Autodesk Fusion 360 part; units mm, degrees
sketch "Sketch1" plane through (0, 0, 0) normal (0, 0, 1) x (1, 0, 0)
  line L0 (18.75, -9.5) -> (-18.75, -9.5)
  line L1 (-18.75, -9.5) -> (-18.75, 9.5)
  line L2 (-18.75, 9.5) -> (18.75, 9.5)
  line L3 (18.75, 9.5) -> (18.75, -9.5)
  line L4 (18.75, -9.5) -> (-18.75, 9.5) construction
  line L5 (-18.75, -9.5) -> (18.75, 9.5) construction
  line L6 (0, 9.5) -> (0, -9.5) construction
  line L7 (12.7, 9.5) -> (12.7, -9.5) construction
  line L8 (-12.7, 9.5) -> (-12.7, -9.5) construction
  line L9 (-5.1, -7.1) -> (3, -7.1)
  line L10 (-3.1043, 7.1) -> (4.9957, 7.1)
  line L11 (-5.1, -7.1) -> (-3.1043, 7.1)
  line L12 (3, -7.1) -> (4.9957, 7.1)
  line L13 (-1.9308, 5.75) -> (3.4427, 5.75)
  line L14 (1.8265, -5.75) -> (3.4427, 5.75)
  line L15 (-3.547, -5.75) -> (1.8265, -5.75)
  line L16 (-3.547, -5.75) -> (-1.9308, 5.75)
  line L17 (-17.8, -7.1) -> (-15.8043, 7.1)
  line L18 (-16.247, -5.75) -> (-14.6308, 5.75)
  line L19 (-17.8, -7.1) -> (-9.7, -7.1)
  line L20 (-16.247, -5.75) -> (-10.8735, -5.75)
  line L21 (-10.8735, -5.75) -> (-9.2573, 5.75)
  line L22 (-9.7, -7.1) -> (-7.7043, 7.1)
  line L23 (-14.6308, 5.75) -> (-9.2573, 5.75)
  line L24 (-15.8043, 7.1) -> (-7.7043, 7.1)
  line L25 (7.6, -7.1) -> (9.5957, 7.1)
  line L26 (9.153, -5.75) -> (10.7692, 5.75)
  line L27 (7.6, -7.1) -> (15.7, -7.1)
  line L28 (9.153, -5.75) -> (14.5265, -5.75)
  line L29 (14.5265, -5.75) -> (16.1427, 5.75)
  line L30 (15.7, -7.1) -> (17.6957, 7.1)
  line L31 (10.7692, 5.75) -> (16.1427, 5.75)
  line L32 (9.5957, 7.1) -> (17.6957, 7.1)
  dimension "d1" = 37.5
  dimension "d2" = 19
  dimension "d3" = 12.7
  dimension "d4" = 12.7
  dimension "d5" = 8.1
  dimension "d6" = 3
  dimension "d7" = 2.4
  dimension "d8" = 8.1
  dimension "d9" = 2.4
  dimension "d10" = 82
  dimension "d11" = -1.35
  dimension "d14" = 12.7
  dimension "d15" = 0
extrude "Extrude1" add sketch "Sketch1" against normal blind 8 contours L0 L1 L2 L3 | L9 L10 L11 L12 | L13 L14 L15 L16 | L17 L19 L22 L24 | L18 L20 L21 L23 | L25 L27 L30 L32 | L26 L28 L29 L31
extrude "Extrude2" cut sketch "Sketch1" against normal blind 0.5 contours L9 L10 L11 L12 | L17 L19 L22 L24 | L25 L27 L30 L32
sketch "Sketch2" plane through (0, -9.5, 0) normal (0, -1, 0) x (1, 0, 0)
  line L0 (18.75, 0) -> (-18.75, 0)
  line L1 (-18.75, 0) -> (-18.75, -8)
  line L2 (-18.75, -8) -> (18.75, -8)
  line L3 (18.75, -8) -> (18.75, 0)
  line L4 (-17.25, -8) -> (-16.25, -7)
  line L5 (-16.25, -7) -> (16.25, -7)
  line L6 (16.25, -7) -> (17.25, -8)
  dimension "d20" = 1
  dimension "d21" = 1.5
  dimension "d22" = 1.5
  dimension "d23" = 45
extrude "Extrude3" cut sketch "Sketch2" against normal up to surface (19 mm away) contours L2 L4 L5 L6
sketch "Sketch3" plane through (-18.75, 0, 0) normal (-1, 0, 0) x (0, -1, 0)
  line L0 (9.5, 0) -> (-9.5, 0)
  line L1 (-9.5, 0) -> (-9.5, -8)
  line L2 (-9.5, -8) -> (9.5, -8)
  line L3 (9.5, -8) -> (9.5, 0)
  line L4 (-8, -8) -> (-7, -7)
  line L5 (-7, -7) -> (7, -7)
  line L6 (7, -7) -> (8, -8)
  dimension "d26" = 45
  dimension "d27" = 1
  dimension "d28" = 1.5
  dimension "d29" = 1.5
extrude "Extrude4" cut sketch "Sketch3" against normal up to surface (37.5 mm away) contours L2 L4 L5 L6
sketch "Sketch4" plane through (0, 0, -7) normal (0, 0, -1) x (1, 0, 0)
  line L0 (16.25, 7) -> (16.25, 9.5)
  line L1 (16.25, 9.5) -> (-16.25, 9.5)
  line L2 (-16.25, 9.5) -> (-16.25, 7)
  line L3 (-16.25, 7) -> (-18.75, 7)
  line L4 (-18.75, 7) -> (-18.75, -7)
  line L5 (-18.75, -7) -> (-16.25, -7)
  line L6 (-16.25, -7) -> (-16.25, -9.5)
  line L7 (-16.25, -9.5) -> (16.25, -9.5)
  line L8 (16.25, -9.5) -> (16.25, -7)
  line L9 (16.25, -7) -> (18.75, -7)
  line L10 (18.75, -7) -> (18.75, 7)
  line L11 (18.75, 7) -> (16.25, 7)
  circle A0 centre (-6.35, 7.62) radius 0.255
  circle A1 centre (-3.81, 7.62) radius 0.255
  circle A2 centre (-1.27, 7.62) radius 0.255
  circle A3 centre (1.27, 7.62) radius 0.255
  circle A4 centre (3.81, 7.62) radius 0.255
  circle A5 centre (6.35, 7.62) radius 0.255
  circle A6 centre (-6.35, -7.62) radius 0.255
  circle A7 centre (-3.81, -7.62) radius 0.255
  circle A8 centre (-1.27, -7.62) radius 0.255
  circle A9 centre (1.27, -7.62) radius 0.255
  circle A10 centre (3.81, -7.62) radius 0.255
  circle A11 centre (6.35, -7.62) radius 0.255
  dimension "d32" = 0.51
  dimension "d33" = 6.35
  dimension "d34" = 7.62
  dimension "d37" = 12.7
  dimension "d38" = -15.24
extrude "Extrude5" add sketch "Sketch4" along normal blind 4 contours A0 | A1 | A2 | A3 | A4 | A5 | A6 | A7 | A8 | A9 | A10 | A11
equation "d4 = d3"
equation "d7 = ( ( 19 - 14.2 ) / 2 ) * 1 mm"
equation "d8 = d5"
equation "d9 = d7"
equation "d22 = d21"
equation "d34 = ( 15.24 / 2 ) * 1 mm"
The listing builds one solid part. Answer for the finished solid, in the listing's coordinates (mm). A direction names the side the tool comes from. Round coordinates to 2 decimals unless told otherwise and drop trailing zeros. Loops run counter-clockwise (first coordinate to the right, second up) from the corner with the lowest first, then second, coordinate; pieces in that order, holes last. Notation, with made-up numbers: (61.5, 35.25) - (101.5, 35.25) arc R21 cw to (101.5, 58.25) - close; hole circle Ø10 at (-31, -5.5). An arc over 180 degrees is marked (long way). Return JSON: item names as keys, results as strings. Group by question number.
1. The part is cut by section D-D on x = 10. Determine the outline of the cut face in (y, z), then the cut area to 3 significant figures.
2. This flat-tipped pin is pushed along its axis until it touches: P1, Ø1.6, axis at x = -18, y = -8.5, coming from the -Z side. Where does it stop, or does it pass through?
3. Consider probe 1 along Z at (x, y) = (11, -5.25); probe 2 along Z at (x, y) = (-15, 5.75). Determine where each line is inside the solid, lowest interval first.
4. Which of the six approach directions +Z, -Z, +X, -X, +Y, -Y give full straight-line access (tool end or side, diameter ignored) to faces 1 (the flat face through (-17.8, -7.5, -7.5)), 2 (the flat face through (-15.45, -0.08, -0.25)), 3 (the flat face through (16.74, 8.51, -7.49)), 4 (the flat face through (0, 0, -7)), 5 (the flat face through (0, 9.5, -4))?
5. The mould has two halves that part along X. Classify faces 6 (the flat face through (-2.75, -0.08, -0.25)), 7 (the flat face through (0, -9.5, -4)), 8 (the flat face through (18.75, 0, -4)): pulls with the +X half, pulls with the -X half, needs draft (parallel to the pull), parting line crosses it, or undercut.
6. The part is cut by section A-A on y = -8.5. Determine the outline of the cut face in (x, z).
7. The part is cut by section C-C on y = -5. Determine the outline of the cut face in (x, z), then the cut area to 3 significant figures.
8. The part is cut by section B-B on x = 0. Determine the outline of the cut face in (y, z).
Resolved:
{
 "1": {"outline": "(-9.5, -7) - (9.5, -7) - (9.5, 0) - (7.1, 0) - (7.1, -0.5) - (0.28, -0.5) - (0.28, 0) - (-5.75, 0) - (-5.75, -0.5) - (-7.1, -0.5) - (-7.1, 0) - (-9.5, 0) - close", "area": "129 mm²"},
 "2": {"P1": "stops at z = -8"},
 "3": {"probe 1": "z = -7 to 0", "probe 2": "z = -7 to -0.5"},
 "4": {"face 1": "-Z, -X", "face 2": "+Z", "face 3": "-Z, +Y, -Y", "face 4": "-Z", "face 5": "+Z, -Z, +X, -X, +Y"},
 "5": {"face 6": "undercut", "face 7": "needs draft", "face 8": "pulls with the +X half"},
 "6": {"outline": "(-18.75, -8) - (-17.25, -8) - (-16.25, -7) - (16.25, -7) - (17.25, -8) - (18.75, -8) - (18.75, 0) - (-18.75, 0) - close"},
 "7": {"outline": "(-18.75, -7) - (18.75, -7) - (18.75, 0) - (16, 0) - (16, -0.5) - (14.63, -0.5) - (14.63, 0) - (9.26, 0) - (9.26, -0.5) - (7.9, -0.5) - (7.9, 0) - (3.3, 0) - (3.3, -0.5) - (1.93, -0.5) - (1.93, 0) - (-3.44, 0) - (-3.44, -0.5) - (-4.8, -0.5) - (-4.8, 0) - (-9.4, 0) - (-9.4, -0.5) - (-10.77, -0.5) - (-10.77, 0) - (-16.14, 0) - (-16.14, -0.5) - (-17.5, -0.5) - (-17.5, 0) - (-18.75, 0) - close", "area": "258 mm²"},
 "8": {"outline": "(-9.5, -7) - (9.5, -7) - (9.5, 0) - (7.1, 0) - (7.1, -0.5) - (5.75, -0.5) - (5.75, 0) - (-5.75, 0) - (-5.75, -0.5) - (-7.1, -0.5) - (-7.1, 0) - (-9.5, 0) - close"}
}
